```python
from build123d import *

# Parameters (mm, degrees)
SKETCH_1_W                     = 306
SKETCH_1_H                     = 47
EXTRUDE_1_DEPTH                = 3
CUT_EXTRUDE_START              = 3
SKETCH_1_4_W                   = 306
SKETCH_1_4_H                   = 6
CUT_EXTRUDE_1_DEPTH            = 1
M3X0_5_3_D                     = 2.5
M3X0_5_3_DEPTH                 = 8.5
M3X0_5_3_CBORE_D               = 3
M3X0_5_3_CBORE_DEPTH           = 6
M3X0_5_3_TIP                   = 0.751075774
M3X0_5_3_ON_FACE_2_D           = 2.5
M3X0_5_3_ON_FACE_2_DEPTH       = 8.5
M3X0_5_3_ON_FACE_2_CBORE_D     = 3
M3X0_5_3_ON_FACE_2_CBORE_DEPTH = 6
M3X0_5_3_ON_FACE_2_TIP         = 0.751075774
PATTERN_LINEAR_1_COUNT         = 11
PATTERN_LINEAR_1_PITCH         = 30
SKETCH_7_R                     = 1.25
CUT_EXTRUDE_2_DEPTH            = 155.910458106


with BuildPart() as part:
    # ｽｹｯﾁ1 → ﾎﾞｽ - 押し出し1 (new, symmetric)
    with BuildSketch(Plane.XY):
        Rectangle(SKETCH_1_W, SKETCH_1_H)
    extrude(amount=EXTRUDE_1_DEPTH, both=True)

    # ｽｹｯﾁ1<4> → ｶｯﾄ - 押し出し1 (cut)
    with BuildSketch(Plane.XY.offset(CUT_EXTRUDE_START)):
        with Locations((0, -20.5)):
            Rectangle(SKETCH_1_4_W, SKETCH_1_4_H)
    extrude(amount=-CUT_EXTRUDE_1_DEPTH, mode=Mode.SUBTRACT)

    # ｽｹｯﾁ2 → M3 すきま穴1 (revolve, cut)
    with BuildSketch(Plane(origin=(-150, -20.5, -3), x_dir=(0, 1, 0), z_dir=(1, 0, 0))):
        Polygon((0, 0), (0, 6.96137699), (1.6, 6), (1.6, 0), align=None)
    hole_wizard_m3_1 = revolve(axis=Axis((-150, -20.5, -9.35), (0, 0, 1)), mode=Mode.SUBTRACT)

    # M3x0.5 ねじ穴3
    with Locations(Plane(origin=(-153, 13.5, 0), x_dir=(0, 0, -1), z_dir=(-1, 0, 0))):
        with Locations((0, 0), (0, 28)):
            CounterBoreHole(M3X0_5_3_D / 2, M3X0_5_3_CBORE_D / 2, M3X0_5_3_CBORE_DEPTH, depth=M3X0_5_3_DEPTH)
            with Locations((0, 0, -(M3X0_5_3_DEPTH + M3X0_5_3_TIP / 2))):  # 118° drill point
                Cone(0, M3X0_5_3_D / 2, M3X0_5_3_TIP, mode=Mode.SUBTRACT)

    # M3x0.5 ねじ穴3 on face 2
    with Locations(Plane(origin=(153, 13.5, 0), x_dir=(0, 0, 1), z_dir=(1, 0, 0))):
        with Locations((0, 0), (0, 28)):
            CounterBoreHole(M3X0_5_3_ON_FACE_2_D / 2, M3X0_5_3_ON_FACE_2_CBORE_D / 2, M3X0_5_3_ON_FACE_2_CBORE_DEPTH, depth=M3X0_5_3_ON_FACE_2_DEPTH)
            with Locations((0, 0, -(M3X0_5_3_ON_FACE_2_DEPTH + M3X0_5_3_ON_FACE_2_TIP / 2))):  # 118° drill point
                Cone(0, M3X0_5_3_ON_FACE_2_D / 2, M3X0_5_3_ON_FACE_2_TIP, mode=Mode.SUBTRACT)

    # ｽｹｯﾁ6 → M3x0.5 ねじ穴2 (revolve, cut)
    with BuildSketch(Plane(origin=(-150, 23.5, 0), x_dir=(0, 0, 1), z_dir=(1, 0, 0))):
        Polygon((0, 0), (0, 9.251075774), (1.25, 8.5), (1.25, 6), (1.5, 6), (1.5, 0), align=None)
    m3x0_5_2 = revolve(axis=Axis((-150, 29.85, 0), (0, -1, 0)), mode=Mode.SUBTRACT)

    # 直線ﾊﾟﾀｰﾝ1: M3 すきま穴1, M3x0.5 ねじ穴2 ×11
    with Locations(*[(i * PATTERN_LINEAR_1_PITCH, 0, 0) for i in range(1, PATTERN_LINEAR_1_COUNT)]):
        add(hole_wizard_m3_1, mode=Mode.SUBTRACT)
        add(m3x0_5_2, mode=Mode.SUBTRACT)

    # ｽｹｯﾁ7 → ｶｯﾄ - 押し出し2 (cut, through all)
    with BuildSketch(Plane(origin=(0, 0, -3), x_dir=(-1, 0, 0), z_dir=(0, 0, -1))):
        with Locations((37.5, 13.5)):
            Circle(SKETCH_7_R)
        with Locations((75.5, 13.5)):
            Circle(SKETCH_7_R)
        with Locations((37.5, -13.5)):
            Circle(SKETCH_7_R)
        with Locations((75.5, -13.5)):
            Circle(SKETCH_7_R)
        with Locations((-19, 13.5)):
            Circle(SKETCH_7_R)
        with Locations((19, 13.5)):
            Circle(SKETCH_7_R)
        with Locations((-19, -13.5)):
            Circle(SKETCH_7_R)
        with Locations((19, -13.5)):
            Circle(SKETCH_7_R)
        with Locations((-75.5, 13.5)):
            Circle(SKETCH_7_R)
        with Locations((-37.5, 13.5)):
            Circle(SKETCH_7_R)
        with Locations((-75.5, -13.5)):
            Circle(SKETCH_7_R)
        with Locations((-37.5, -13.5)):
            Circle(SKETCH_7_R)
        with BuildLine():
            Line((69, -9), (44, -9))
            ThreePointArc((44, -9), (35, 0), (44, 9))
            Line((44, 9), (69, 9))
            ThreePointArc((69, 9), (78, 0), (69, -9))
        make_face()
        with BuildLine():
            Line((12.5, -9), (-12.5, -9))
            ThreePointArc((-12.5, -9), (-21.5, 0), (-12.5, 9))
            Line((-12.5, 9), (12.5, 9))
            ThreePointArc((12.5, 9), (21.5, 0), (12.5, -9))
        make_face()
        with BuildLine():
            Line((-44, -9), (-69, -9))
            ThreePointArc((-69, -9), (-78, 0), (-69, 9))
            Line((-69, 9), (-44, 9))
            ThreePointArc((-44, 9), (-35, 0), (-44, -9))
        make_face()
    extrude(amount=-CUT_EXTRUDE_2_DEPTH, mode=Mode.SUBTRACT)


solid = part.part
```
Check sheet for the modelled part. Datum: model origin and axes. Units: mm. A direction names the side the tool comes from. Round coordinates to 2 decimals unless told otherwise and drop trailing zeros. Write each loop counter-clockwise with the first axis right and the second up, starting at its lowest first coordinate (ties: lowest second). Pieces come first, ordered by that corner, then holes. Notation, with made-up numbers: M 2.25,62 L 55.25,62 A27 ccw 55.25,97 Z; hole C -2,-31.75 d9. An arc over 180 degrees is marked long. Write item = value, one per line. Start each with the question number.
1. Scan lines: line 1 (X direction, y = 6.5, z = -2.15); line 2 (Z direction, x = 120, y = 16); line 3 (X direction, y = -6, z = 1.8). Record each from-to range of solid material in increasing order. Write a range as [from, to].
2. Section check B-B, the plane x = 80.5. Record the cut outline in (y, z).
3. Release check for a two-part mould opening along Y. For faces 1 (the flat face through (-2, 23.5, 0)), 2 (the flat face through (153, 0, 0)), 3 (the cylindrical face through (35, 0, 0)) record: pulls with the +Y half, pulls with the -Y half, needs draft (parallel to the pull), parting line crosses it, or undercut.
4. Gauge pin test, flat ends, axial feed: pin 1 (0.9 mm diameter, centred on x = 60, z = 0.5, fed in from +Y); pin 2 (3.5 mm diameter, centred on x = 60, y = -20.5, fed in from +Z); pin 3 (3 mm diameter, centred on x = 13, y = 8, fed in from +Z); pin 4 (0.9 mm diameter, centred on y = 13, z = 0, fed in from -X). Record the tip position at first contact, or that the pin passes through.
5. Tool access check on faces 4 (the flat face through (-2, -20, 2)), 5 (the flat face through (57, 9, 0)), 6 (the flat face through (-2, 12, 3)). Record the directions out of +Z, -Z, +X, -X, +Y, -Y that give a thin tool (end or side, any length) a straight path to the whole face; none if there is none.
6. Section check A-A, the plane y = 1. Record the cut outline in (x, z).
Results found:
q1.line_1 = [-153, -75.22], [-37.78, -18.72], [18.72, 37.78], [75.22, 153]
q1.line_2 = [-3, -1.25], [1.25, 3]
q1.line_3 = [-153, -75.71], [-37.29, -19.21], [19.21, 37.29], [75.71, 153]
q2.outline = M -23.5,-3 L 23.5,-3 L 23.5,3 L -17.5,3 L -17.5,2 L -23.5,2 Z
q3.face_1 = pulls with the +Y half
q3.face_2 = needs draft
q3.face_3 = undercut
q4.pin_1 = 14.82
q4.pin_2 = 2
q4.pin_3 = 3
q4.pin_4 = -144.32
q5.face_4 = +Z, +X, -X, -Y
q5.face_5 = +Z, -Z
q5.face_6 = +Z, +X, -X, +Y, -Y
q6.outline = M -153,-3 L -77.94,-3 L -77.94,3 L -153,3 Z; M -35.06,-3 L -21.44,-3 L -21.44,3 L -35.06,3 Z; M 21.44,-3 L 35.06,-3 L 35.06,3 L 21.44,3 Z; M 77.94,-3 L 153,-3 L 153,3 L 77.94,3 Z
